Input: part model. Units: mm. Frame: model coordinates. A direction names the side the tool comes from. Coordinates: 2 decimals unless noted, no trailing zeros. Order: outer loops, then holes, each group sorted by start corner. A loop starts at its lowest first (then second) coordinate and runs counter-clockwise, first axis right, second up. Notation, with made-up numbers: (47.5, 15) -> (67.5, 15) arc R8 cw to (67.5, 28) -> close; hole circle Ø6 at (86.5, 3.25). An arc over 180 degrees is marked (long way). One line per question, with ' | ' between items.
```python
from build123d import *

# Parameters (mm, degrees)
F0_W     = 200
F0_H     = 200
F1_DEPTH = 5
F2_W     = 200
F2_H     = 5
F3_DEPTH = 60
F4_R     = 25
F5_DEPTH = 25
F6_R     = 20
F7_DEPTH = 25


with BuildPart() as f1:
    # F0 (on Front) → F1 (new body)
    with BuildSketch(Plane.XZ):
        with Locations((44.733446, 57.222639)):
            Rectangle(F0_W, F0_H)
    extrude(amount=F1_DEPTH)

    # F2 (on face) → F3 (join)
    with BuildSketch(Plane.XZ.offset(5)):
        with Locations((44.733446, -40.277361)):
            Rectangle(F2_W, F2_H)
    extrude(amount=F3_DEPTH)

    # F4 (on face) → F5 (join)
    with BuildSketch(Plane.XZ.offset(5)):
        with Locations((0, 112.222639)):
            Circle(F4_R)
    extrude(amount=F5_DEPTH)

    # F6 (on face) → F7 (cut)
    with BuildSketch(Plane.XZ.offset(30)):
        with Locations((0, 112.222639)):
            Circle(F6_R)
    extrude(amount=-F7_DEPTH, mode=Mode.SUBTRACT)


solid = f1.part
```
1. Cut plane C-C, the plane z = 83. Return loops of the section in (x, y).
Recorded:
outline: (-55.27, -5) -> (144.73, -5) -> (144.73, 0) -> (-55.27, 0) -> close
2. Cut plane A-A, the plane x = 0. Return loops of the section in (y, z), and give its area (3 significant figures).
Recorded:
outline: (-65, -42.78) -> (0, -42.78) -> (0, 157.22) -> (-5, 157.22) -> (-5, 137.22) -> (-30, 137.22) -> (-30, 132.22) -> (-5, 132.22) -> (-5, 92.22) -> (-30, 92.22) -> (-30, 87.22) -> (-5, 87.22) -> (-5, -37.78) -> (-65, -37.78) -> close | area: 1,550 mm^2
3. Pin query (flat end, axial travel): pin 1 Ø15 at (x, z) = (0.5, 118.5) entering from -Y; pin 2 Ø1.5 at (x, z) = (14, 26) entering from +Y; pin 3 Ø1.5 at (x, y) = (60.5, -23) entering from +Z; pin 4 Ø8 at (y, z) = (-23.5, 96.5) entering from +X. Return the tip coordinate at first contact, or that it passes through.
Recorded:
pin 1: stops at y = -5 | pin 2: stops at y = 0 | pin 3: stops at z = -37.78 | pin 4: stops at x = 22.08
4. Access query for faces 4 (the face through (43, -2, 157.223)), 5 (the face through (-11.2, -30, 129)), 6 (the face through (10.75, -17.68, 129.09)). Directions: +Z, -Z, +X, -X, +Y, -Y. A direction counts if a zero-diameter tool reaches every point of the face in a straight line with its end or side. Return the directions, or none.
Recorded:
face 4: +Z, +X, -X, +Y, -Y | face 5: +Z, +X, -X, -Y | face 6: -Y
5. Mould query, pull axis X, two halves, no side actions, for faces 1 (the face through (0, -5, 113)), 2 (the face through (43, -35, -37.777)), 3 (the face through (-5.42, -17.325, 87.817)). Classes: released by +X, released by -X, zero draft, split by the parting line, or undercut.
Recorded:
face 1: undercut | face 2: zero draft | face 3: split by the parting line
6. Ray query, line 1 (Z direction, x = 0, y = -20); line 2 (Z direction, x = 15, y = -5.5); line 3 (Y direction, x = 37, z = 60). Return the intervals inside material, ascending. Write a range as [from, to].
Recorded:
line 1: z = [-42.78, -37.78], [87.22, 92.22], [132.22, 137.22] | line 2: z = [-42.78, -37.78], [92.22, 98.99], [125.45, 132.22] | line 3: y = [-5, 0]
7. Cut plane B-B, the plane y = -21. Return loops of the section in (x, z).
Recorded:
outline: (-55.27, -42.78) -> (144.73, -42.78) -> (144.73, -37.78) -> (-55.27, -37.78) -> close; circle Ø50 at (0, 112.22); hole circle Ø40 at (0, 112.22)
8. Cut plane D-D, the plane y = -39. Return loops of the section in (x, z), and give its area (3 significant figures).
Recorded:
outline: (-55.27, -42.78) -> (144.73, -42.78) -> (144.73, -37.78) -> (-55.27, -37.78) -> close | area: 1,000 mm^2
